```python
from build123d import *

# Parameters (mm, degrees)
F0_W     = 6.35
F0_H     = 12.7
F1_DEPTH = 12.7
F2_W     = 3.5
F2_H     = 1
F3_DEPTH = 6.35
F4_R     = 1
F5_DEPTH = 12.701


with BuildPart() as f1:
    # F0 (on Top) → F1 (new body)
    with BuildSketch(Plane.XY):
        with Locations((3.175, 6.35)):
            Rectangle(F0_W, F0_H)
    extrude(amount=F1_DEPTH)

    # F2 (on face) → F3 (join)
    with BuildSketch(Plane.XY.offset(12.7)):
        with Locations((3.175, 9.025)):
            Rectangle(F2_W, F2_H)
        with Locations((3.175, 3.675)):
            Rectangle(F2_W, F2_H)
    extrude(amount=F3_DEPTH)

    # F4 (on face) → F5 (cut, through all)
    with BuildSketch(Plane(origin=(0, 12.7, 0), x_dir=(-1, 0, 0), z_dir=(0, 1, 0))):
        with Locations((-3.175, 6.35)):
            Circle(F4_R)
    extrude(amount=-F5_DEPTH, mode=Mode.SUBTRACT)


solid = f1.part
```
Work out the finished part from the listing and answer in its coordinate system (mm). A direction names the side the tool comes from. Coordinates: 2 decimals unless noted, no trailing zeros. Write each loop counter-clockwise with the first axis right and the second up, starting at its lowest first coordinate (ties: lowest second). Pieces come first, ordered by that corner, then holes. Notation, with made-up numbers: (38.5, 78) - (72.5, 78) arc R23 ccw to (72.5, 91) - close; hole circle Ø2 at (70, -38). An arc over 180 degrees is marked (long way). Answer as a JSON object with one key per item and string values.
Q1. Given pin 1 Ø1 at (x, z) = (3.5, 17) entering from -Y (3 decimals); pin 2 Ø1.1 at (y, z) = (9, 16) entering from +X (3 decimals); pin 3 Ø1.8 at (x, z) = (3, 16) entering from +Y (3 decimals), each flat-ended and moving along its own axis, determine where each tip first touches the part or whether it passes through.
Results list:
{"pin 1": "stops at y = 3.175", "pin 2": "stops at x = 4.925", "pin 3": "stops at y = 9.525"}
Q2. Find section C-C (y = 12.25). Write down the section's boundary in (x, z) (3 decimals).
Results list:
{"outline": "(0, 0) - (6.35, 0) - (6.35, 12.7) - (0, 12.7) - close; hole circle Ø2 at (3.175, 6.35)"}
Q3. Which of the six approach directions +Z, -Z, +X, -X, +Y, -Y give full straight-line access (tool end or side, diameter ignored) to faces 4 (the flat face through (3, 9.525, 16)), 5 (the flat face through (1.425, 4, 16)), 6 (the flat face through (4.925, 4, 16)), 7 (the flat face through (3, 4.175, 16)), 8 (the flat face through (3, 3.175, 16))?
Results list:
{"face 4": "+Z, +X, -X, +Y", "face 5": "+Z, -X, +Y, -Y", "face 6": "+Z, +X, +Y, -Y", "face 7": "+Z, +X, -X", "face 8": "+Z, +X, -X, -Y"}
Q4. Find section A-A (z = 6.35). Write down the section's boundary in (x, y) (3 decimals), plus the area to 3 significant figures.
Results list:
{"outline": "(0, 0) - (2.175, 0) - (2.175, 12.7) - (0, 12.7) - close; (4.175, 0) - (6.35, 0) - (6.35, 12.7) - (4.175, 12.7) - close", "area": "55.2 mm^2"}
Q5. Find section D-D (x = 5.5). Write down the section's boundary in (y, z), plus the area to 3 significant figures.
Results list:
{"outline": "(0, 0) - (12.7, 0) - (12.7, 12.7) - (0, 12.7) - close", "area": "161 mm^2"}
Q6. For a pull along Y with two mould halves and no side action, classify faces 1 (the flat face through (3, 6, 0)), 2 (the flat face through (5, 0, 6)), 3 (the flat face through (3, 8.525, 16)) as pulls with the +Y half, pulls with the -Y half, needs draft (parallel to the pull), parting line crosses it, or undercut.
Results list:
{"face 1": "needs draft", "face 2": "pulls with the -Y half", "face 3": "undercut"}
Q7. Consider L1, parallel to Y at x = 1.5, z = 16.25 (3 decimals); L2, parallel to Z at x = 4.5, y = 2.25; L3, parallel to Z at x = 4, y = 2. Determine where each line is inside the solid, lowest interval first. Write a range as from..to.
Results list:
{"L1": "y = 3.175..4.175, 8.525..9.525", "L2": "z = 0..12.7", "L3": "z = 0..5.78, 6.92..12.7"}
Q8. Find section B-B (y = 3.75). Write down the section's boundary in (x, z) (3 decimals).
Results list:
{"outline": "(0, 0) - (6.35, 0) - (6.35, 12.7) - (4.925, 12.7) - (4.925, 19.05) - (1.425, 19.05) - (1.425, 12.7) - (0, 12.7) - close; hole circle Ø2 at (3.175, 6.35)"}
